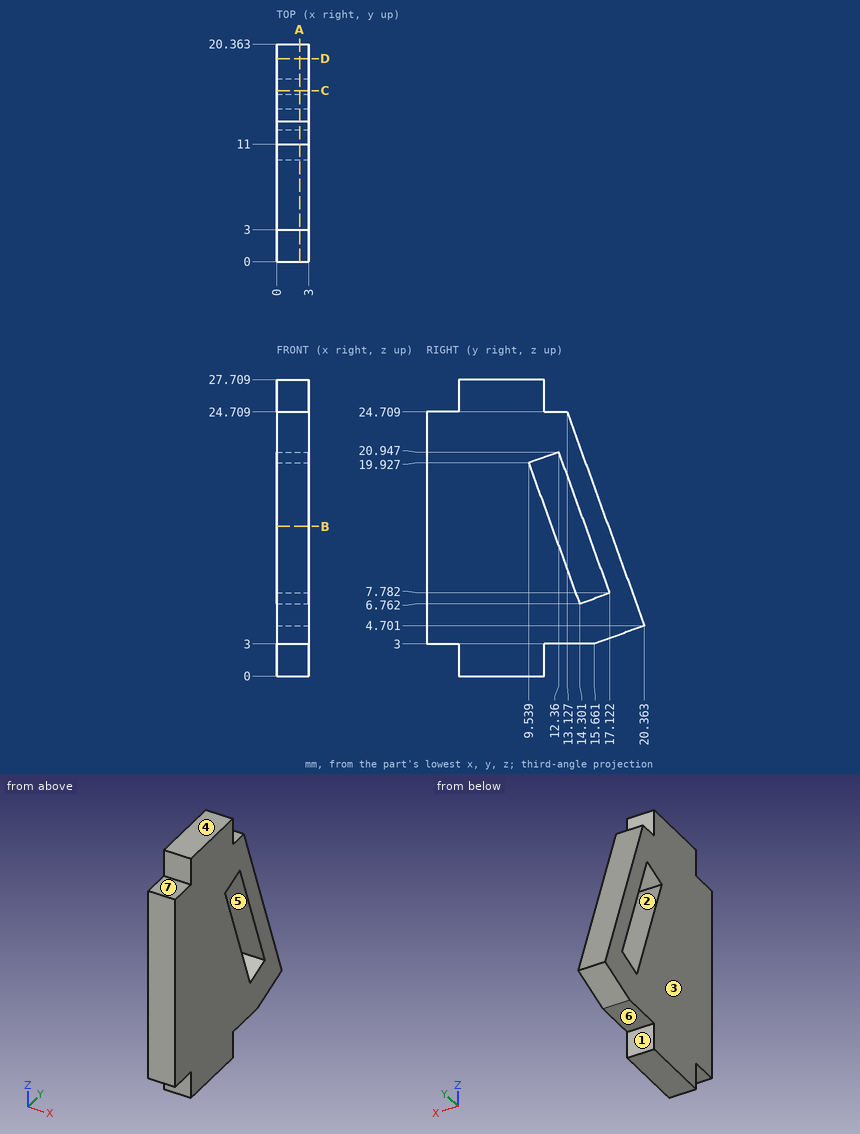
Verification items for this drawing (mm, ordinates from the low corner). A direction names the side the tool comes from. Round coordinates to 2 decimals unless told otherwise and drop trailing zeros. Loops run counter-clockwise (first coordinate to the right, second up) from the corner with the lowest first, then second, coordinate; pieces in that order, holes last. Notation, with made-up numbers: (-29.75, -0.5) -> (-7.75, -0.5) arc R17 cw to (-7.75, 32.5) -> close; hole circle Ø4 at (12.25, 39.5). An arc over 180 degrees is marked (long way). Write item = value, one per line. Start each with the question number.
1) Sectioned sample at D-D, the plane y = 19. Record the cut outline in (x, z).
2) Sectioned sample at C-C, the plane y = 16. Record the cut outline in (x, z) (1 decimal).
3) Release check for a two-part mould opening along Y. For the marked faces 1, 2 and 3 record: released by +Y, released by -Y, zero draft, split by the parting line, or undercut.
4) Thickness scan on probe 1 along Y at (x, z) = (0.7, 14); probe 2 along Y at (x, z) = (2.45, 13.5) (1 decimal); probe 3 along Y at (x, z) = (2.2, 26.5). Record the ranges inside material, lowest first.
5) Sectioned sample at A-A, the plane x = 2.15. Record the cut outline in (y, z).
6) Gauge pin test, flat ends, axial feed: pin 1 Ø0.9 at (x, z) = (2, 1.5) entering from -Y; pin 2 Ø0.9 at (x, z) = (1.5, 1.5) entering from +Y; pin 3 Ø1.5 at (x, y) = (1.5, 14.5) entering from -Z. Record the tip position at first contact, or that the pin passes through.
7) Sectioned sample at B-B, the plane z = 14. Record the cut outline in (x, y).
8) Set-up check for the marked faces 4, 5, 6 and 7: record each of +Z, -Z, +X, -X, +Y, -Y from which the full face is reachable in a straight line by a thin tool's end or side.
Results are:
q1.outline = (0, 4.21) -> (3, 4.21) -> (3, 8.47) -> (0, 8.47) -> close
q2.outline = (0, 3.1) -> (3, 3.1) -> (3, 7.4) -> (0, 7.4) -> close; (0, 10.9) -> (3, 10.9) -> (3, 16.8) -> (0, 16.8) -> close
q3.face_1 = released by +Y
q3.face_2 = undercut
q3.face_3 = zero draft
q4.probe_1 = 0 to 11.68, 14.87 to 17
q4.probe_2 = 0 to 11.9, 15.1 to 17.2
q4.probe_3 = 3 to 11
q5.outline = (0, 3) -> (3, 3) -> (3, 0) -> (11, 0) -> (11, 3) -> (15.66, 3) -> (20.36, 4.7) -> (13.13, 24.71) -> (11, 24.71) -> (11, 27.71) -> (3, 27.71) -> (3, 24.71) -> (0, 24.71) -> close; hole (9.54, 19.93) -> (14.3, 6.76) -> (17.12, 7.78) -> (12.36, 20.95) -> close
q6.pin_1 = 3
q6.pin_2 = 11
q6.pin_3 = 3
q7.outline = (0, 0) -> (3, 0) -> (3, 11.68) -> (0, 11.68) -> close; (0, 14.87) -> (3, 14.87) -> (3, 17) -> (0, 17) -> close
q8.face_4 = +Z, +X, -X, +Y, -Y
q8.face_5 = +X, -X
q8.face_6 = -Z, +X, -X, +Y
q8.face_7 = +Z, +X, -X, -Y
